Answer from the drawing. Dimensions are ordinates in mm from the lowest x, y and z of the part. A direction names the side the tool comes from. Round coordinates to 2 decimals unless told otherwise and drop trailing zeros.
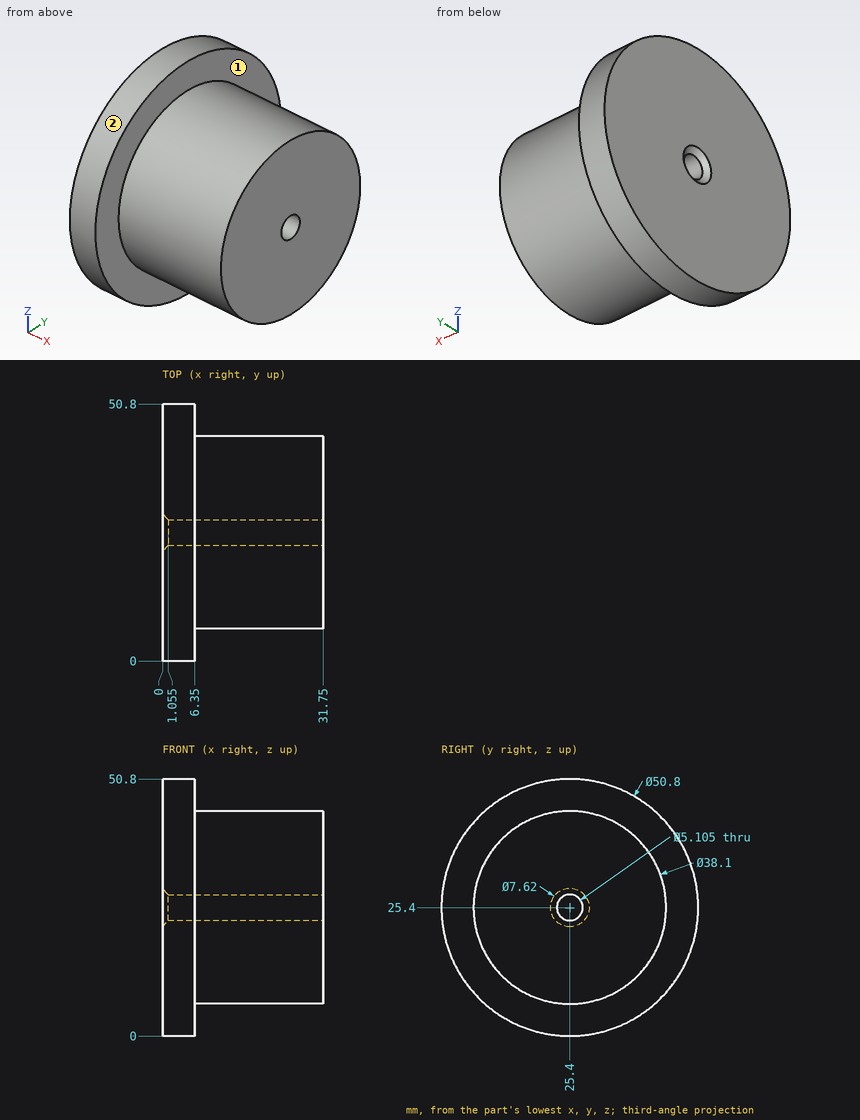
Item 1: For the marked faces 1 and 2, determine the directions among +Z, -Z, +X, -X, +Y, -Y from which every point of the face is accessible in a straight line to the end or side of a thin tool.
Item 2: Straight lines are drawn through the part: line 1 (Z direction, x = 6.5, y = 25.5); line 2 (Z direction, x = 17, y = 25) (1 decimal). For each, find the intervals that lie inside material, in ascending order.
Item 3: Each of these flat-tipped pins is pushed along its axis until it touches: P1, Ø6, axis at y = 25.4, z = 25.4, coming from the -X side; P2, Ø2, axis at x = 22, z = 14, coming from the +Y side; P3, Ø10, axis at x = 11, y = 36.5, coming from the -Z side. Where does it stop, or does it pass through?
Answer below:
1. face 1: +X
1. face 2: +X, -X
2. line 1: z = 6.35 to 22.85, 27.95 to 44.45
2. line 2: z = 6.4 to 22.9, 27.9 to 44.4
3. P1: stops at x = 0.68
3. P2: stops at y = 41.36
3. P3: stops at z = 1.75
